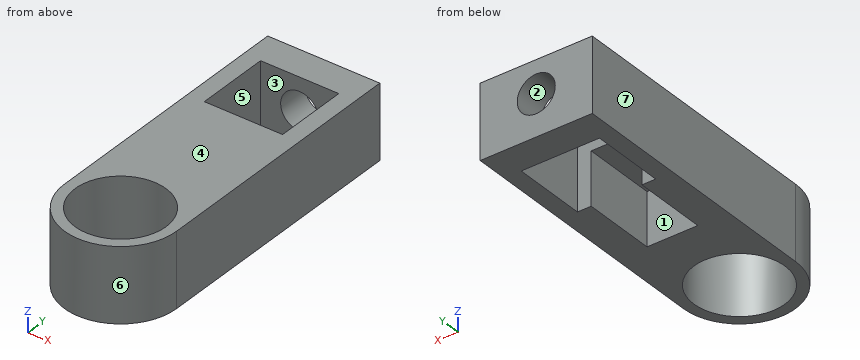
Autodesk Fusion 360 part; units mm, degrees
sketch "Sketch1" plane through (0, 0, 0) normal (0, 0, 1) x (1, 0, 0)
  circle A0 centre (0, 0) radius 5.461
  line L0 (-6.731, 0) -> (-6.731, 32.131)
  line L1 (6.731, 0) -> (6.731, 32.131)
  line L2 (4.699, 19.431) -> (-4.699, 19.431)
  line L3 (-4.699, 19.431) -> (-4.699, 28.321)
  line L4 (-4.699, 28.321) -> (4.699, 28.321)
  line L5 (4.699, 28.321) -> (4.699, 19.431)
  line L6 (4.699, 19.431) -> (-4.699, 28.321) construction
  line L7 (-4.699, 19.431) -> (4.699, 28.321) construction
  line L8 (-6.731, 32.131) -> (6.731, 32.131)
  arc A1 (-6.731, 0) -> (6.731, 0) centre (0, 0) ccw
  point P0 (0, 23.876)
  point P1 (0, 6.731)
  dimension "d1" = 10.922
  dimension "d2" = 13.462
  dimension "d5" = 9.398
  dimension "d6" = 8.89
  dimension "d7" = 12.7
  dimension "d8" = 3.81
extrude "Extrude1" add sketch "Sketch1" along normal blind 8.89
sketch "Sketch3" plane through (0, 32.131, 0) normal (0, 1, 0) x (-1, 0, 0)
  line L0 (-6.731, 0) -> (6.731, 0)
  line L1 (6.731, 0) -> (6.731, 8.89)
  line L2 (6.731, 8.89) -> (-6.731, 8.89)
  line L3 (-6.731, 8.89) -> (-6.731, 0)
  line L4 (0, 8.89) -> (0, 7.239)
  circle A0 centre (0, 4.953) radius 2.286
  dimension "d12" = 1.651
  dimension "d13" = 4.572
extrude "Extrude2" cut sketch "Sketch3" against normal blind 5.842 contours A0
sketch "Sketch4" plane through (0, 0, 8.89) normal (0, 0, 1) x (-1, 0, 0)
  circle A0 centre (0, 0) radius 5.461
  line L0 (4.699, -28.321) -> (-4.699, -28.321)
  line L1 (-4.699, -28.321) -> (-4.699, -19.431)
  line L2 (-4.699, -19.431) -> (4.699, -19.431)
  line L3 (4.699, -19.431) -> (4.699, -28.321)
  line L4 (6.731, -32.131) -> (6.731, 0)
  arc A1 (6.731, 0) -> (-6.731, 0) centre (0, 0) ccw
  line L5 (-6.731, 0) -> (-6.731, -32.131)
  line L6 (-6.731, -32.131) -> (6.731, -32.131)
sketch "Sketch5" plane through (0, 0, 0) normal (0, 0, 1) x (1, 0, 0)
  line L0 (-3.048, 20.6883) -> (3.048, 20.6883)
  line L1 (3.048, 20.6883) -> (3.048, 10.6044)
  line L2 (3.048, 10.6044) -> (-3.048, 10.6044)
  line L3 (-3.048, 10.6044) -> (-3.048, 20.6883)
  point P0 (0, 10.6044)
  dimension "d18" = 6.096
extrude "Extrude3" cut sketch "Sketch5" along normal blind 6.35
Input: part model. Units: mm. Frame: model coordinates. Face numbers are marked on the shaded views. A direction names the side the tool comes from. Coordinates: 2 decimals unless noted, no trailing zeros. Order: outer loops, then holes, each group sorted by start corner. A loop starts at its lowest first (then second) coordinate and runs counter-clockwise, first axis right, second up. Notation, with made-up numbers: M 79.5,-9 L 120.5,-9 A17 cw 120.5,10 Z; hole C -37,87 d2. An arc over 180 degrees is marked long. Write item = value, one per line. Start each with the question number.
(1) Section D-D on z = 4.5. Output: boundary loops of the cut face in (x, y), and give its area (3 significant figures).
(2) Section C-C on z = 8. Output: boundary loops of the cut face in (x, y), and give its area (3 significant figures).
(3) Section A-A on x = 0. Output: boundary loops of the cut face in (y, z).
(4) Section B-B on y = 25. Output: boundary loops of the cut face in (x, z), and give its area (3 significant figures).
(5) Reachability of the marked faces 1, 2, 3 and 4 from +Z, -Z, +X, -X, +Y, -Y: full face, straight path, thin tool, end or side. Return the list, or none.
(6) First-contact query: P1, Ø2.5, axis at x = -1.5, z = 4, coming from the +Y side; P2, Ø1.8, axis at x = -0.5, y = 15, coming from the -Z side; P3, Ø5, axis at x = 5, z = 7, coming from the -Y side; P4, Ø6.5, axis at x = 0, y = 0, coming from the -Z side. Flat tips, straight axial feed; report the tip coordinate or a pass-through.
(7) Line query: line 1 along Y through (x, z) = (0, 6.5); line 2 along X through (y, z) = (17, 5.5); line 3 along Y through (x, z) = (-0.25, 4.25). Output: solid intervals per line, ascending. Write a range as [from, to].
(8) Pull-direction query (Y, two-part tool) for the marked faces 5, 6 and 7; classes: released by +Y, released by -Y, zero draft, split by the parting line, or undercut.
Result set:
q1.outline = M -6.73,0 A6.73 ccw 6.73,0 L 6.73,32.13 L 2.24,32.13 L 2.24,28.32 L 4.7,28.32 L 4.7,19.43 L 3.05,19.43 L 3.05,10.6 L -3.05,10.6 L -3.05,19.43 L -4.7,19.43 L -4.7,28.32 L -2.24,28.32 L -2.24,32.13 L -6.73,32.13 Z; hole C 0,0 d10.92
q1.area = 256 mm²
q2.outline = M -6.73,0 A6.73 ccw 6.73,0 L 6.73,32.13 L -6.73,32.13 Z; hole C 0,0 d10.92; hole M -4.7,19.43 L 4.7,19.43 L 4.7,28.32 L -4.7,28.32 Z
q2.area = 326 mm²
q3.outline = M -6.73,0 L -5.46,0 L -5.46,8.89 L -6.73,8.89 Z; M 5.46,0 L 10.6,0 L 10.6,6.35 L 19.43,6.35 L 19.43,8.89 L 5.46,8.89 Z; M 28.32,0 L 32.13,0 L 32.13,2.67 L 28.32,2.67 Z; M 28.32,7.24 L 32.13,7.24 L 32.13,8.89 L 28.32,8.89 Z
q4.outline = M -6.73,0 L -4.7,0 L -4.7,8.89 L -6.73,8.89 Z; M 4.7,0 L 6.73,0 L 6.73,8.89 L 4.7,8.89 Z
q4.area = 36.1 mm²
q5.face_1 = -Z
q5.face_2 = +Y
q5.face_3 = +Z, -Z
q5.face_4 = +Z, +X, -X, +Y, -Y
q6.P1 = 32.13
q6.P2 = 6.35
q6.P3 = -6.25
q6.P4 = through
q7.line_1 = [-6.73, -5.46], [5.46, 19.43]
q7.line_2 = [-6.73, -3.05], [3.05, 6.73]
q7.line_3 = [-6.73, -5.46], [5.46, 10.6]
q8.face_5 = undercut
q8.face_6 = released by -Y
q8.face_7 = zero draft
